from build123d import *

# Parameters (mm, degrees)
F0_R     = 2
F0_R_2   = 8.85
F1_DEPTH = 6


# Not quite as in the source:
# - a feature names something its author has since deleted; it is built from what else it names


with BuildPart() as f1:
    # F0 (on Top) → F1 (new body)
    with BuildSketch(Plane.XY):
        Polygon((-20, 15.6), (-20, 12), (-20, -12), (18, -12), (18, -9), (45.65, -9), (45.65, -12), (50, -12), (50, 15.6), (45.65, 15.6), (45.65, 12), (16.15, 12), (16.15, 15.6), (3.15, 15.6), (3.15, 13.4), (5, 13.4), (5, 12), (-5, 12), (-5, 13.4), (-3.15, 13.4), (-3.15, 15.6), align=None)
        with Locations((-15, -7)):
            Circle(F0_R, mode=Mode.SUBTRACT)
        Circle(F0_R_2, mode=Mode.SUBTRACT)
        with Locations((15, -7)):
            Circle(F0_R, mode=Mode.SUBTRACT)
        with Locations((45, 1.8)):
            Circle(F0_R, mode=Mode.SUBTRACT)
    extrude(amount=F1_DEPTH)


solid = f1.part
Model file for the job. Use its own axes, mm. A direction names the side the tool comes from. Give positions to 0.01 mm unless a question says otherwise; leave off trailing zeros. Order: outer loops, then holes, each group sorted by start corner. A loop starts at its lowest first (then second) coordinate and runs counter-clockwise, first axis right, second up. Notation, with made-up numbers: M 42,36.5 L 83,36.5 A36 ccw 83,75.5 Z; hole C -9,88.5 d4. An arc over 180 degrees is marked long. Write item = value, one per line.
Q1. Flat gauge pin, fed straight in: pin 1 (3 mm diameter, centred on x = 35, z = 2.5, fed in from -Y). Where does the tip first touch, or does it go through?
Derived:
pin_1 = -9
Q2. Two-plate mould, pull along X, no slides. Class faces 1 (the flat face through (-20, 2, 3)), 2 (the flat face through (15, 2, 6)), 3 (the cylindrical face through (43.002, 1.888, 2.958)), 4 (the flat face through (5, 13, 3)): pulls with the +X half, pulls with the -X half, needs draft (parallel to the pull), parting line crosses it, or undercut.
Derived:
face_1 = pulls with the -X half
face_2 = needs draft
face_3 = undercut
face_4 = undercut
Q3. Cut at A-A, the plane x = 15. List the corners of the cut face in (y, z), then the cut area to 3 significant figures.
Derived:
outline = M -12,0 L -9,0 L -9,6 L -12,6 Z; M -5,0 L 15.6,0 L 15.6,6 L -5,6 Z
area = 142 mm2
Q4. Cut at D-D, the plane y = -8. List the corners of the cut face in (x, z), then the cut area to 3 significant figures.
Derived:
outline = M -20,0 L -16.73,0 L -16.73,6 L -20,6 Z; M -13.27,0 L -3.78,0 L -3.78,6 L -13.27,6 Z; M 3.78,0 L 13.27,0 L 13.27,6 L 3.78,6 Z; M 16.73,0 L 50,0 L 50,6 L 16.73,6 Z
area = 333 mm2
Q5. Drill centre lines: line 1 (X direction, y = -6.75, z = 0.95); line 2 (Y direction, x = 45, z = 4.45); line 3 (X direction, y = 13, z = 0.5). Where is each one in solid material? Low to high. Write a range as [from, to].
Derived:
line_1 = [-20, -16.98], [-13.02, -5.72], [5.72, 13.02], [16.98, 50]
line_2 = [-9, -0.2], [3.8, 12]
line_3 = [-20, -5], [5, 16.15], [45.65, 50]
Q6. Cut at C-C, the plane y = -2.5. List the corners of the cut face in (x, z).
Derived:
outline = M -20,0 L -8.49,0 L -8.49,6 L -20,6 Z; M 8.49,0 L 50,0 L 50,6 L 8.49,6 Z
Q7. Tool access for faces 5 (the flat face through (-4, 13.4, 3)), 6 (the flat face through (31, 12, 3)), 7 (the flat face through (45.65, -10, 3)), 8 (the flat face through (-1, -12, 3)): list every direction of +Z, -Z, +X, -X, +Y, -Y with a clear straight run to the whole face (end or side of a thin tool).
Derived:
face_5 = +Z, -Z
face_6 = +Z, -Z, +Y
face_7 = +Z, -Z, -Y
face_8 = +Z, -Z, +X, -X, -Y
Q8. Cut at B-B, the plane z = 5.3. List the corners of the cut face in (x, y).
Derived:
outline = M -20,-12 L 18,-12 L 18,-9 L 45.65,-9 L 45.65,-12 L 50,-12 L 50,15.6 L 45.65,15.6 L 45.65,12 L 16.15,12 L 16.15,15.6 L 3.15,15.6 L 3.15,13.4 L 5,13.4 L 5,12 L -5,12 L -5,13.4 L -3.15,13.4 L -3.15,15.6 L -20,15.6 Z; hole C -15,-7 d4; hole C 0,0 d17.7; hole C 15,-7 d4; hole C 45,1.8 d4
